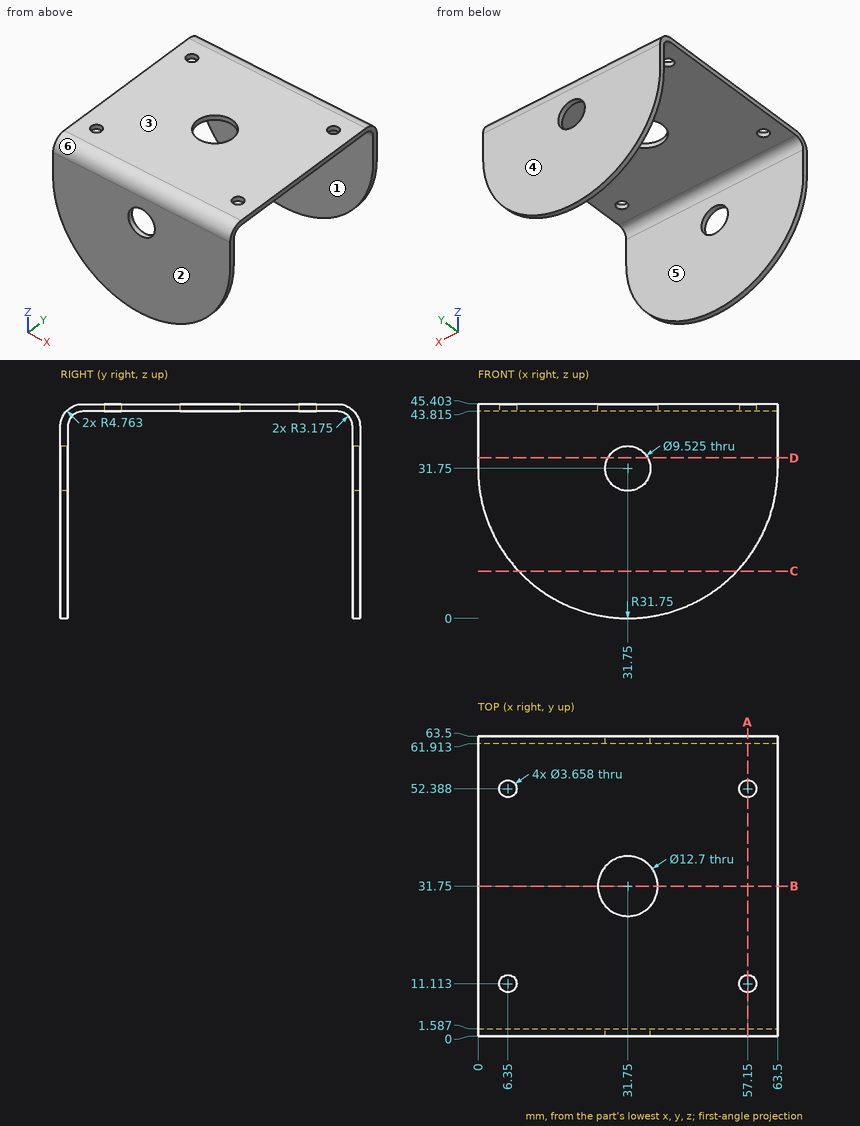
Here's the drawing with two shaded views (mm, measured from the low corner). I have some questions. A direction names the side the tool comes from. Round coordinates to 2 decimals unless told otherwise and drop trailing zeros. Order: outer loops, then holes, each group sorted by start corner. A loop starts at its lowest first (then second) coordinate and runs counter-clockwise, first axis right, second up. Notation, with made-up numbers: M 45,68 L 52,68 A32 cw 52,106 Z; hole C 19,26 d10. An arc over 180 degrees is marked long. Use CSV: the item, a comma, the result in double quotes.
1) I want a section at A-A (x = 57.15). Count the separate pieces of the cut face and the enclosed holes in it.
Taken from the geometry:
separate pieces,"3"
enclosed holes,"0"
2) I'm going to push a flat-ended pin straight in: P1, Ø4, axis at x = 57.15, y = 11.11, coming from the -Z side (1 decimal). Where does the tip first touch, or does it pass through?
Taken from the geometry:
P1,"z = 43.8"
3) I want a section at B-B (y = 31.75). List the corners of the cut face in (x, z) for me (1 decimal).
Taken from the geometry:
outline,"M 0,43.8 L 25.4,43.8 L 25.4,45.4 L 0,45.4 Z; M 38.1,43.8 L 63.5,43.8 L 63.5,45.4 L 38.1,45.4 Z"
4) I want a section at D-D (z = 34). List the corners of the cut face in (x, y) for me.
Taken from the geometry:
outline,"M 0,0 L 27.55,0 L 27.55,1.59 L 0,1.59 Z; M 0,61.91 L 27.55,61.91 L 27.55,63.5 L 0,63.5 Z; M 35.95,0 L 63.5,0 L 63.5,1.59 L 35.95,1.59 Z; M 35.95,61.91 L 63.5,61.91 L 63.5,63.5 L 35.95,63.5 Z"
5) If we mould it in two halves opening along Y, with no side actions, what happens to the marked faces 3, 4, 5 and 6? For each: pulls with the +Y half, pulls with the -Y half, needs draft (parallel to the pull), parting line crosses it, or undercut.
Taken from the geometry:
face 3,"needs draft"
face 4,"pulls with the +Y half"
face 5,"undercut"
face 6,"pulls with the -Y half"
6) I need wall thicknesses on line 1 along Y through (x, z) = (36.5, 33); line 2 along Y through (x, z) = (6.35, 44.75) (1 decimal); line 3 along Y through (x, z) = (57.15, 44.6) (1 decimal). Which ranges of each line are inside material? Lowest first, please. Write a range as [from, to].
Taken from the geometry:
line 1,"[0, 1.59], [61.91, 63.5]"
line 2,"[2.4, 9.3], [12.9, 50.6], [54.2, 61.1]"
line 3,"[2.1, 9.3], [12.9, 50.6], [54.2, 61.4]"
7) I want a section at C-C (z = 10). List the corners of the cut face in (x, y) for me.
Taken from the geometry:
outline,"M 8.62,0 L 54.88,0 L 54.88,1.59 L 8.62,1.59 Z; M 8.62,61.91 L 54.88,61.91 L 54.88,63.5 L 8.62,63.5 Z"
8) On a 3-axis mill with a long thin cutter (end or side, diameter ignored), from which of +Z, -Z, +X, -X, +Y, -Y can I reach the whole of each face in a straight line? I mean the marked faces 1 and 2. Say none if no direction works.
Taken from the geometry:
face 1,"-Z, +X, -X"
face 2,"+Z, -Z, +X, -X, -Y"
